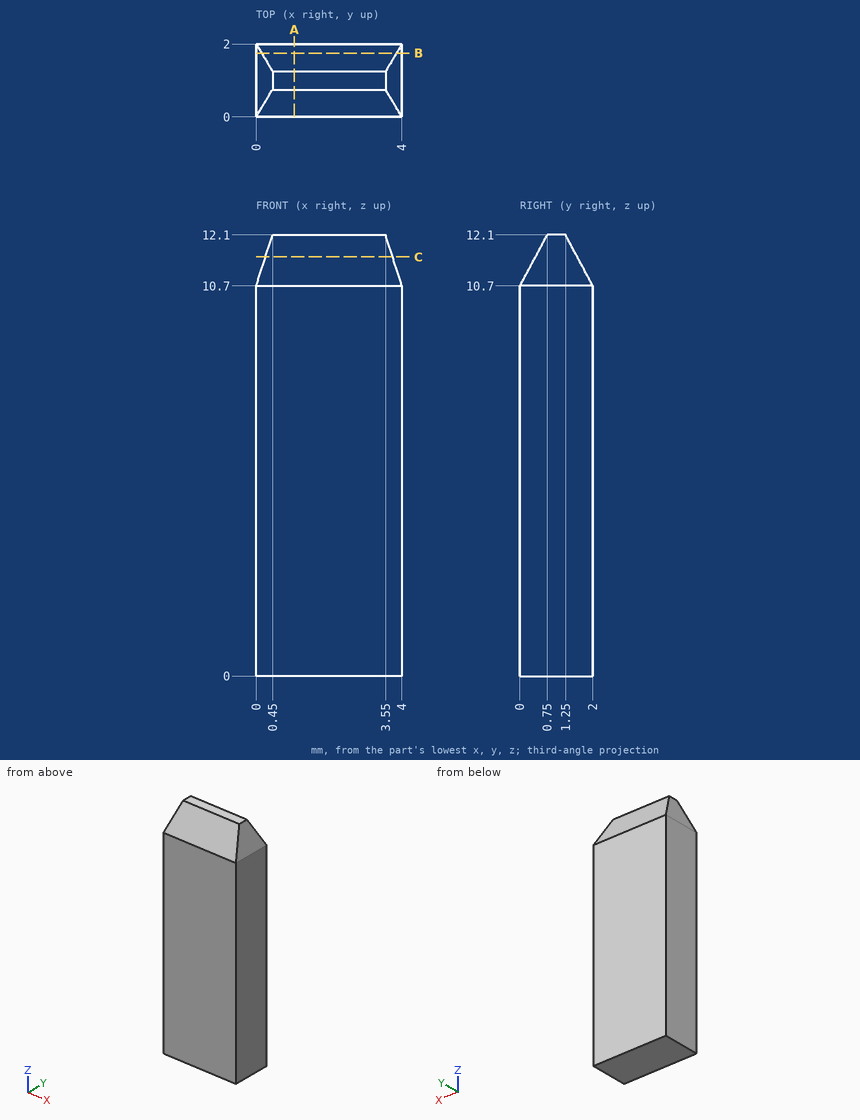
Source: three-view drawing plus pictorial views. Frame: mm from the lowest corner of the part. Coordinates: 2 decimals unless noted, no trailing zeros. Write each loop counter-clockwise with the first axis right and the second up, starting at its lowest first coordinate (ties: lowest second). Pieces come first, ordered by that corner, then holes. Notation, with made-up numbers: (17, 83) - (51, 83) arc R31 ccw to (51, 114) - close; hole circle Ø2 at (10.25, -22). An arc over 180 degrees is marked (long way). Answer as a JSON object with one key per item and string values.
Q1. Section query A-A, the plane x = 1.05. Output: boundary loops of the cut face in (y, z), plus the area to 4 significant figures.
Ans:
{"outline": "(0, 0) - (2, 0) - (2, 10.7) - (1.25, 12.1) - (0.75, 12.1) - (0, 10.7) - close", "area": "23.15 mm2"}
Q2. Section query B-B, the plane y = 1.75. Output: boundary loops of the cut face in (x, z), plus the area to 3 significant figures.
Ans:
{"outline": "(0, 0) - (4, 0) - (4, 10.7) - (3.85, 11.17) - (0.15, 11.17) - (0, 10.7) - close", "area": "44.6 mm2"}
Q3. Section query C-C, the plane z = 11.5. Output: boundary loops of the cut face in (x, y).
Ans:
{"outline": "(0.26, 0.43) - (3.74, 0.43) - (3.74, 1.57) - (0.26, 1.57) - close"}
Q4. Material intervals for line 1 (Z direction, x = 2.6, y = 1.55); line 2 (Z direction, x = 0.85, y = 0.3), sorted ascending. Write a range as [from, to].
Ans:
{"line 1": "z = [0, 11.54]", "line 2": "z = [0, 11.26]"}
